Autodesk Inventor part; units mm, degrees
ref_plane "YZ Plane" through (0, 0, 0) normal (1, 0, 0) x (0, 1, 0)
ref_plane "XZ Plane" through (0, 0, 0) normal (0, 1, 0) x (-1, 0, 0)
ref_plane "XY Plane" through (0, 0, 0) normal (0, 0, 1) x (1, 0, 0)
sketch "草圖1" plane through (0, 0, 0) normal (0, 0, 1) x (1, 0, 0)
  line L0 (-5, 15) -> (5, 15)
  line L1 (5, 15) -> (5, 0)
  line L2 (5, 0) -> (-5, 0)
  line L3 (-5, 0) -> (-5, 15)
  line L4 (-4, 0) -> (4, 0)
  line L5 (4, 0) -> (4, -3)
  line L6 (4, -3) -> (-4, -3)
  line L7 (-4, -3) -> (-4, 0)
  circle A0 centre (0, 10) radius 3.5
  point P0 (0, 0)
  point P1 (0, 0)
  dimension "d0" = 3
  dimension "d1" = 8
  dimension "d2" = 15
  dimension "d3" = 7
  dimension "d4" = 5
  dimension "d5" = 10
extrude "擠出1" add sketch "草圖1" along normal blind 3
properties part number "land"
The listing builds one solid part. Answer for the finished solid, in the listing's coordinates (mm). A direction names the side the tool comes from. Coordinates: 2 decimals unless noted, no trailing zeros. Loops run counter-clockwise (first coordinate to the right, second up) from the corner with the lowest first, then second, coordinate; pieces in that order, holes last. Notation, with made-up numbers: M -26,-35 L 13,-35 A22 ccw 13,-15 Z; hole C 8.5,44 d4. An arc over 180 degrees is marked long. Answer in a Markdown table with one row per item.
1) Find section A-A (x = 0). Determine the outline of the cut face in (y, z), then the cut area to 3 significant figures.
Answers below:
| item | result |
|---|---|
| outline | M -3,0 L 6.5,0 L 6.5,3 L -3,3 Z; M 13.5,0 L 15,0 L 15,3 L 13.5,3 Z |
| area | 33.0 mm^2 |
2) Find section B-B (y = 7.25). Determine the outline of the cut face in (x, z), then the cut area to 3 significant figures.
Answers below:
| item | result |
|---|---|
| outline | M -5,0 L -2.17,0 L -2.17,3 L -5,3 Z; M 2.17,0 L 5,0 L 5,3 L 2.17,3 Z |
| area | 17.0 mm^2 |
3) Find the intervals of material crossed by probe 1 along Y at (x, z) = (0, 1.4); probe 2 along X at (y, z) = (7.25, 1.55); probe 3 along X at (y, z) = (11.25, 0.7), in increasing order.
Answers below:
| item | result |
|---|---|
| probe 1 | -3 to 6.5, 13.5 to 15 |
| probe 2 | -5 to -2.17, 2.17 to 5 |
| probe 3 | -5 to -3.27, 3.27 to 5 |
4) Which of the six approach directions +Z, -Z, +X, -X, +Y, -Y give full straight-line access (tool end or side, diameter ignored) to faces 1 (the flat face through (4, -1, 1)), 2 (the flat face through (0, 6, 3)), 3 (the flat face through (-4, -2, 1))?
Answers below:
| item | result |
|---|---|
| face 1 | +Z, -Z, +X, -Y |
| face 2 | +Z, +X, -X, +Y, -Y |
| face 3 | +Z, -Z, -X, -Y |
5) Given pin 1 (3 mm diameter, centred on x = 0, y = 12.5, fed in from +Z); pin 2 (0.9 mm diameter, centred on y = -1.5, z = 1.5, fed in from -X); pin 3 (0.8 mm diameter, centred on x = -4.5, z = 1, fed in from -Y), each flat-ended and moving along its own axis, determine where each tip first touches the part or whether it passes through.
Answers below:
| item | result |
|---|---|
| pin 1 | z = 3 |
| pin 2 | x = -4 |
| pin 3 | y = 0 |
6) Find section D-D (x = 4.5). Determine the outline of the cut face in (y, z).
Answers below:
| item | result |
|---|---|
| outline | M 0,0 L 15,0 L 15,3 L 0,3 Z |
7) Find section C-C (z = 2.65). Determine the outline of the cut face in (x, y).
Answers below:
| item | result |
|---|---|
| outline | M -5,0 L -4,0 L -4,-3 L 4,-3 L 4,0 L 5,0 L 5,15 L -5,15 Z; hole C 0,10 d7 |
8) Determine the mould class of faces 4 (the cylindrical face through (-0.759, 13.417, 1.479)), 5 (the flat face through (5, 8, 1)), 6 (the flat face through (0, -3, 1)) for opening direction X: released by +X, released by -X, zero draft, split by the parting line, or undercut.
Answers below:
| item | result |
|---|---|
| face 4 | undercut |
| face 5 | released by +X |
| face 6 | zero draft |
